Could you check a few things on this model? Use its own coordinates, in mm. Face numbers are marked on the shaded views. A direction names the side the tool comes from. Round coordinates to 2 decimals unless told otherwise and drop trailing zeros. Loops run counter-clockwise (first coordinate to the right, second up) from the corner with the lowest first, then second, coordinate; pieces in that order, holes last. Notation, with made-up numbers: M -32.5,-35 L 13.5,-35 A7 ccw 13.5,-28 Z; hole C -40,65 d2. An arc over 180 degrees is marked long. One line per item, written item: value. Start each with the question number.
Q1. Please list where these lines run through material, in increasing order: line 1 along Z through (x, y) = (0, -8.4); line 2 along X through (y, z) = (8, 92.5); line 3 along Y through (x, z) = (-16, 30.5).
Q2. Thinking about a two-plate mould opening in Y: for the marked faces 3, 4 and 5, which applies, released by +Y, released by -Y, zero draft, split by the parting line, or undercut?
Q3. Imagine slicing it at A-A (x = 0). Please give me the cut outline in (y, z).
Q4. I'm going to push flat-ended pins straight in: pin 1 Ø8.5 at (x, z) = (0, 71.44) entering from -Y; pin 2 Ø1.5 at (x, z) = (14.5, 11.5) entering from +Y; pin 3 Ø11 at (x, z) = (-4.5, 26) entering from +Y. Where does each tip first touch, or does it pass through?
Q5. Imagine slicing it at B-B (y = -5). Please give me the cut outline in (x, z).
Q6. Imagine slicing it at C-C (z = 40.5). Please give me the cut outline in (x, y) (1 decimal), then the cut area to 3 significant figures.
Q7. Which directions (+Z, -Z, +X, -X, +Y, -Y) give clear straight access to the entire face, cutting with the end or side of a thin tool? Please do the marked faces 1 and 2.
from build123d import *

# Parameters (mm, degrees)
BASE_EXTRUDE_DEPTH = 101.6
HOLE1_START        = -9.0932
HOLE1_OUTLINE_R    = 7.14375
HOLE1_DEPTH        = 2.6924
LPATTERN2_COUNT    = 2
LPATTERN2_PITCH    = 47.625


# Read off the part's stored shape, not the designer's step: Hole1
with BuildPart() as part:
    # Sketch1 → Base-Extrude (new body)
    with BuildSketch(Plane.XY):
        with BuildLine():
            Line((-20.6375, 8.3693), (-20.6375, -6.4008))
            ThreePointArc((-20.6375, -6.4008), (-19.848914298, -8.304614298), (-17.9451, -9.0932))
            Line((-17.9451, -9.0932), (17.9451, -9.0932))
            ThreePointArc((17.9451, -9.0932), (19.848914298, -8.304614298), (20.6375, -6.4008))
            Line((20.6375, -6.4008), (20.6375, 8.3693))
            ThreePointArc((20.6375, 8.3693), (15.875, 13.1318), (11.1125, 8.3693))
            Line((11.1125, 8.3693), (11.1125, 7.33425))
            ThreePointArc((11.1125, 7.33425), (12.4587, 5.98805), (13.8049, 7.33425))
            Line((13.8049, 7.33425), (13.8049, 8.3693))
            ThreePointArc((13.8049, 8.3693), (15.875, 10.4394), (17.9451, 8.3693))
            Line((17.9451, 8.3693), (17.9451, -6.4008))
            Line((17.9451, -6.4008), (-17.9451, -6.4008))
            Line((-17.9451, -6.4008), (-17.9451, 8.3693))
            ThreePointArc((-17.9451, 8.3693), (-15.875, 10.4394), (-13.8049, 8.3693))
            Line((-13.8049, 8.3693), (-13.8049, 7.33425))
            ThreePointArc((-13.8049, 7.33425), (-12.4587, 5.98805), (-11.1125, 7.33425))
            Line((-11.1125, 7.33425), (-11.1125, 8.3693))
            ThreePointArc((-11.1125, 8.3693), (-15.875, 13.1318), (-20.6375, 8.3693))
        make_face()
    extrude(amount=BASE_EXTRUDE_DEPTH)

    # Hole1 outline → Hole1 (cut)
    with BuildSketch(Plane(origin=(0, 0, 0), x_dir=(1, 0, 0), z_dir=(0, 1, 0)).offset(HOLE1_START)):
        with Locations((0, -23.8125)):
            Circle(HOLE1_OUTLINE_R)
    hole1 = extrude(amount=HOLE1_DEPTH, mode=Mode.SUBTRACT)

    # LPattern2: Hole1 ×2
    with Locations(*[(0, 0, i * LPATTERN2_PITCH) for i in range(1, LPATTERN2_COUNT)]):
        add(hole1, mode=Mode.SUBTRACT)


solid = part.part
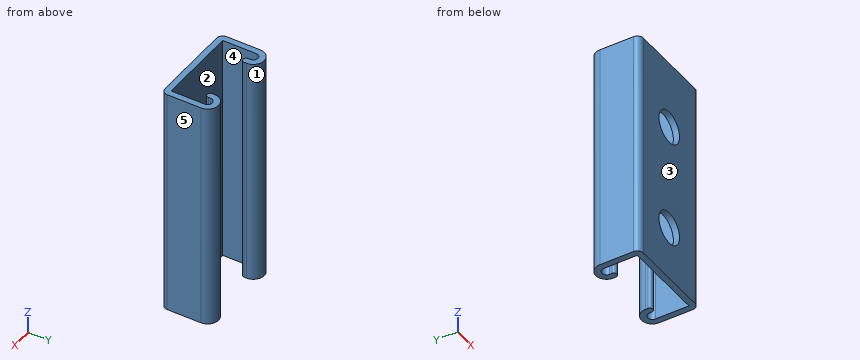
Report:
1. line 1: z = 0 to 16.67, 30.96 to 64.29, 78.58 to 101.6
1. line 2: x = -20.64 to -17.95, -13.8 to -11.11, 11.11 to 13.8, 17.95 to 20.64
1. line 3: y = -9.09 to -6.4, 10.44 to 13.13
2. face 3: released by -Y
2. face 4: undercut
2. face 5: zero draft
3. outline: M -9.09,0 L -6.4,0 L -6.4,16.67 L -9.09,16.67 Z; M -9.09,30.96 L -6.4,30.96 L -6.4,64.29 L -9.09,64.29 Z; M -9.09,78.58 L -6.4,78.58 L -6.4,101.6 L -9.09,101.6 Z
4. pin 1: passes through
4. pin 2: stops at y = 13.09
4. pin 3: stops at y = -6.4
5. outline: M -20.64,0 L -17.95,0 L -17.95,101.6 L -20.64,101.6 Z; M 17.95,0 L 20.64,0 L 20.64,101.6 L 17.95,101.6 Z
6. outline: M -20.6,-6.4 A2.7 ccw -17.9,-9.1 L 17.9,-9.1 A2.7 ccw 20.6,-6.4 L 20.6,8.4 A4.8 ccw 11.1,8.4 L 11.1,7.3 A1.3 ccw 13.8,7.3 L 13.8,8.4 A2.1 cw 17.9,8.4 L 17.9,-6.4 L -17.9,-6.4 L -17.9,8.4 A2.1 cw -13.8,8.4 L -13.8,7.3 A1.3 ccw -11.1,7.3 L -11.1,8.4 A4.8 ccw -20.6,8.4 Z
6. area: 257 mm²
7. face 1: +Z, -Z, +Y
7. face 2: +Z, -Z
